Source: three-view drawing plus pictorial views. Frame: mm from the lowest corner of the part. A direction names the side the tool comes from. Give positions to 0.01 mm unless a question says otherwise; leave off trailing zeros. Loops run counter-clockwise (first coordinate to the right, second up) from the corner with the lowest first, then second, coordinate; pieces in that order, holes last.
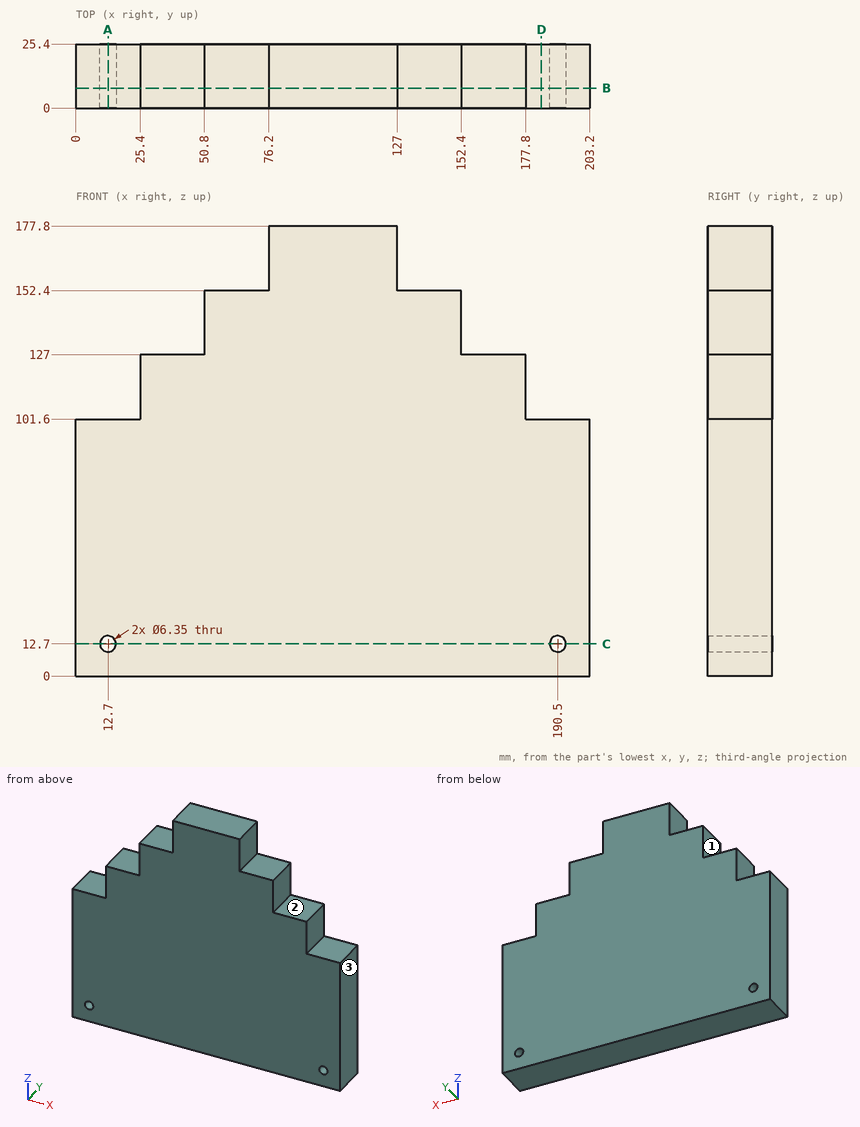
1) Cut plane D-D (x = 184). Return loops of the section in (y, z).
Checks:
outline: (0, 0) - (25.4, 0) - (25.4, 101.6) - (0, 101.6) - close
2) Reachability of the marked faces 1, 2 and 3 from +Z, -Z, +X, -X, +Y, -Y: full face, straight path, thin tool, end or side. Return the list, or none.
Checks:
face 1: +Z, -X, +Y, -Y
face 2: +Z, +X, +Y, -Y
face 3: +Z, -Z, +X, +Y, -Y
3) Cut plane B-B (y = 8). Return loops of the section in (x, z) (3 decimals), and give its area (3 significant figures).
Checks:
outline: (0, 0) - (203.2, 0) - (203.2, 101.6) - (177.8, 101.6) - (177.8, 127) - (152.4, 127) - (152.4, 152.4) - (127, 152.4) - (127, 177.8) - (76.2, 177.8) - (76.2, 152.4) - (50.8, 152.4) - (50.8, 127) - (25.4, 127) - (25.4, 101.6) - (0, 101.6) - close; hole circle Ø6.35 at (12.7, 12.7); hole circle Ø6.35 at (190.5, 12.7)
area: 28,300 mm2
4) Cut plane A-A (x = 12.7). Return loops of the section in (y, z) (3 decimals).
Checks:
outline: (0, 0) - (25.4, 0) - (25.4, 9.525) - (0, 9.525) - close; (0, 15.875) - (25.4, 15.875) - (25.4, 101.6) - (0, 101.6) - close
5) Cut plane C-C (z = 12.7). Return loops of the section in (x, y) (3 decimals), and give its area (3 significant figures).
Checks:
outline: (0, 0) - (9.525, 0) - (9.525, 25.4) - (0, 25.4) - close; (15.875, 0) - (187.325, 0) - (187.325, 25.4) - (15.875, 25.4) - close; (193.675, 0) - (203.2, 0) - (203.2, 25.4) - (193.675, 25.4) - close
area: 4,840 mm2
6) Contact query for flat-ended pins moving along their axis: P1, Ø7.5, axis at y = 12.5, z = 137, coming from the -X side; P2, Ø7.5, axis at x = 188, y = 15.5, coming from the +Z side; P3, Ø5, axis at x = 12.7, z = 12.7, coming from the +Y side; P4, Ø12.5, axis at y = 13, z = 115, coming from the -X side. Output: stop coordinate, or through.
Checks:
P1: stops at x = 50.8
P2: stops at z = 101.6
P3: passes through
P4: stops at x = 25.4
7) Ray query, probe 1 along Z at (x, y) = (190.5, 15) (3 decimals); probe 2 along X at (y, z) = (11, 158); probe 3 along X at (y, z) = (17, 113). Return the intervals inside material, ascending.
Checks:
probe 1: z = 0 to 9.525, 15.875 to 101.6
probe 2: x = 76.2 to 127
probe 3: x = 25.4 to 177.8
